Input: dimensioned drawing with shaded views. Units: mm. Origin: part minimum x, y, z. Give positions to 0.01 mm unless a question says otherwise; leave off trailing zeros. Order: outer loops, then holes, each group sorted by start corner. A loop starts at its lowest first (then second) coordinate and runs counter-clockwise, first axis right, second up. Notation, with made-up numbers: (-33, -39) - (-9, -39) arc R20 cw to (-9, -19) - close; hole circle Ø4 at (6, -12). An arc over 180 degrees is marked (long way). Use a Markdown table: item, result.
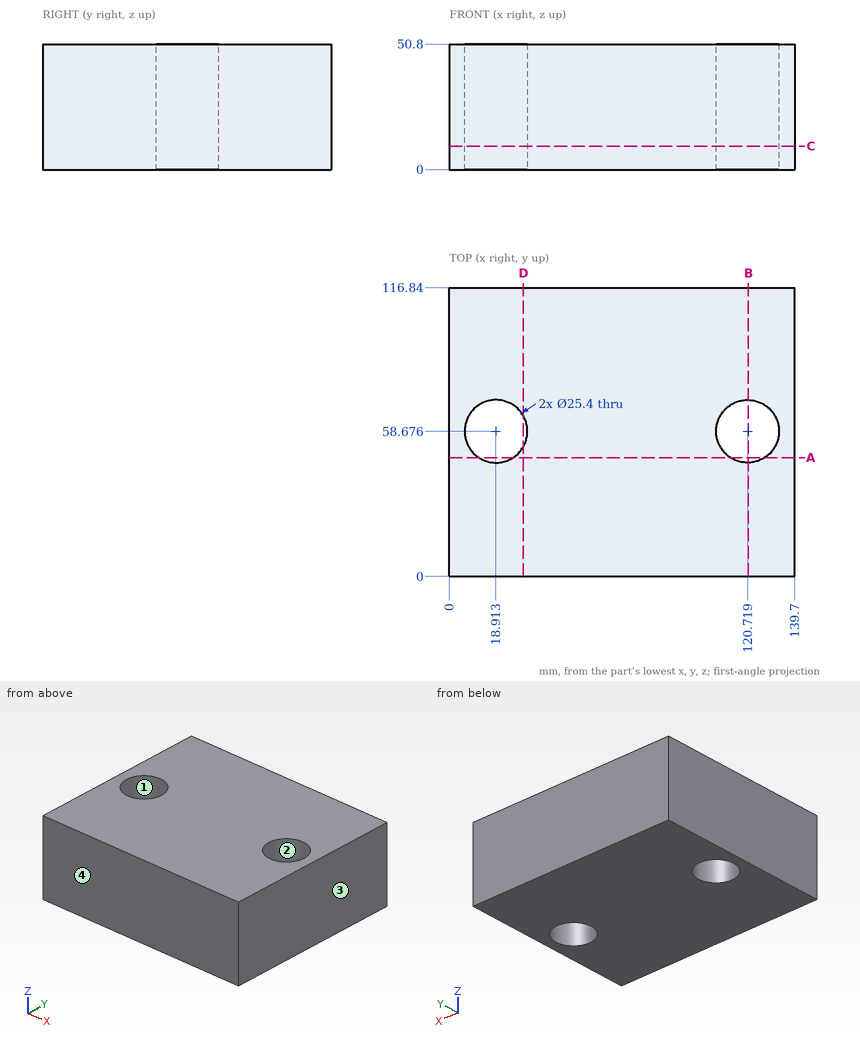
1. Section query C-C (z = 9.5). Return loops of the section in (x, y).
Response:
| item | result |
|---|---|
| outline | (0, 0) - (139.7, 0) - (139.7, 116.84) - (0, 116.84) - close; hole circle Ø25.4 at (18.91, 58.68); hole circle Ø25.4 at (120.72, 58.68) |
2. Mould query, pull axis Y, two halves, no side actions, for the marked faces 1, 2, 3 and 4. Classes: pulls with the +Y half, pulls with the -Y half, needs draft (parallel to the pull), parting line crosses it, or undercut.
Response:
| item | result |
|---|---|
| face 1 | undercut |
| face 2 | undercut |
| face 3 | needs draft |
| face 4 | pulls with the -Y half |
3. Section query B-B (x = 121). Return loops of the section in (y, z).
Response:
| item | result |
|---|---|
| outline | (0, 0) - (45.98, 0) - (45.98, 50.8) - (0, 50.8) - close; (71.37, 0) - (116.84, 0) - (116.84, 50.8) - (71.37, 50.8) - close |
4. Material intervals for line 1 along X through (y, z) = (58.5, 26.5) (1 decimal); line 2 along X through (y, z) = (53.5, 31.5) (1 decimal); line 3 along Y through (x, z) = (128, 14), sorted ascending.
Response:
| item | result |
|---|---|
| line 1 | x = 0 to 6.2, 31.6 to 108, 133.4 to 139.7 |
| line 2 | x = 0 to 7.3, 30.5 to 109.1, 132.3 to 139.7 |
| line 3 | y = 0 to 48.27, 69.08 to 116.84 |
5. Section query D-D (x = 30). Return loops of the section in (y, z).
Response:
| item | result |
|---|---|
| outline | (0, 0) - (52.48, 0) - (52.48, 50.8) - (0, 50.8) - close; (64.87, 0) - (116.84, 0) - (116.84, 50.8) - (64.87, 50.8) - close |
6. Section query A-A (y = 48). Return loops of the section in (x, z) (1 decimal), then the cut area to 3 significant figures.
Response:
| item | result |
|---|---|
| outline | (0, 0) - (12, 0) - (12, 50.8) - (0, 50.8) - close; (25.8, 0) - (113.8, 0) - (113.8, 50.8) - (25.8, 50.8) - close; (127.6, 0) - (139.7, 0) - (139.7, 50.8) - (127.6, 50.8) - close |
| area | 5,700 mm^2 |
